Here's how the part is built. I have some questions about the finished solid (model axes, mm). A direction names the side the tool comes from. Coordinates: 2 decimals unless noted, no trailing zeros. Write each loop counter-clockwise with the first axis right and the second up, starting at its lowest first coordinate (ties: lowest second). Pieces come first, ordered by that corner, then holes.
Item 1: For faces 1 (the face through (-20, 2, 0)), 2 (the face through (0, 2, 17.1)), 3 (the face through (20, 2, 0)), which set-ups out of +Z, -Z, +X, -X, +Y, -Y let a thin tool reach every point of the face, with its end or its side?
Item 2: If we section it at C-C (y = 1.5): Please give me the cut outline in (x, z).
Item 3: If we section it at D-D (z = 20): Please give me the cut outline in (x, y), then the cut area to 3 significant figures.
Item 4: If I drill on line 1 (Z direction, x = -10.5, y = 0.75); line 2 (X direction, y = 2.25, z = -9); line 3 (Z direction, x = -7, y = 3.65), over which ranges is the centre line in solid material (lowest first)?
Item 5: If we section it at B-B (z = 15.5): Please give me the cut outline in (x, y).
Item 6: I'm going to push flat-ended pins straight in: pin 1 Ø1.5 at (x, y) = (-2, 2.5) entering from +Z; pin 2 Ø1.5 at (y, z) = (2.5, 8) entering from -X. Where does each tip first touch, or does it pass through?
Item 7: We'd pull the mould along X, two halves only. Please class faces 4 (the face through (1.435, 0.507, 18.504)), 5 (the face through (0, 4, 0)), 6 (the face through (21.5, 0.5, 0.3)): +X half, -X half, draft (parallel to the pull), parting line (faces both ways), or undercut.
Item 8: If we section it at A-A (x = 4.5): Please give me the cut outline in (y, z).
from build123d import *

# Parameters (mm, degrees)
CROQUIS1_W              = 43
CROQUIS1_H              = 45
SALIENTE_EXTRUIR1_DEPTH = 1
CROQUIS2_W              = 40
CROQUIS2_H              = 34
SALIENTE_EXTRUIR2_DEPTH = 3
CROQUIS3_R              = 0.5
CORTAR_EXTRUIR1_DEPTH   = 2


with BuildPart() as part:
    # Croquis1 → Saliente-Extruir1 (new body)
    with BuildSketch(Plane(origin=(0, 0, 0), x_dir=(1, 0, 0), z_dir=(0, 1, 0))):
        Rectangle(CROQUIS1_W, CROQUIS1_H)
    extrude(amount=SALIENTE_EXTRUIR1_DEPTH)

    # Croquis2 → Saliente-Extruir2 (add)
    with BuildSketch(Plane(origin=(0, 1, 0), x_dir=(1, 0, 0), z_dir=(0, 1, 0))):
        with Locations((0, -0.1)):
            Rectangle(CROQUIS2_W, CROQUIS2_H)
    extrude(amount=SALIENTE_EXTRUIR2_DEPTH)

    # Croquis3 → Cortar-Extruir1 (cut, through all)
    with BuildSketch(Plane(origin=(0, 1, 0), x_dir=(1, 0, 0), z_dir=(0, 1, 0))):
        with Locations((1.5, -19)):
            Circle(CROQUIS3_R)
        with Locations((4.5, -19)):
            Circle(CROQUIS3_R)
        with Locations((7.5, -19)):
            Circle(CROQUIS3_R)
        with Locations((10.5, -19)):
            Circle(CROQUIS3_R)
        with Locations((-10.5, -19)):
            Circle(CROQUIS3_R)
        with Locations((-7.5, -19)):
            Circle(CROQUIS3_R)
        with Locations((-4.5, -19)):
            Circle(CROQUIS3_R)
        with Locations((-1.5, -19)):
            Circle(CROQUIS3_R)
    extrude(amount=-CORTAR_EXTRUIR1_DEPTH, mode=Mode.SUBTRACT)


solid = part.part
Answer list:
1. face 1: +Z, -Z, -X, +Y
1. face 2: +Z, +X, -X, +Y
1. face 3: +Z, -Z, +X, +Y
2. outline: (-20, -16.9) - (20, -16.9) - (20, 17.1) - (-20, 17.1) - close
3. outline: (-21.5, 0) - (21.5, 0) - (21.5, 1) - (-21.5, 1) - close
3. area: 43.0 mm2
4. line 1: z = -22.5 to 18.5, 19.5 to 22.5
4. line 2: x = -20 to 20
4. line 3: z = -16.9 to 17.1
5. outline: (-21.5, 0) - (21.5, 0) - (21.5, 1) - (20, 1) - (20, 4) - (-20, 4) - (-20, 1) - (-21.5, 1) - close
6. pin 1: stops at z = 17.1
6. pin 2: stops at x = -20
7. face 4: undercut
7. face 5: draft
7. face 6: +X half
8. outline: (0, -22.5) - (1, -22.5) - (1, -16.9) - (4, -16.9) - (4, 17.1) - (1, 17.1) - (1, 18.5) - (0, 18.5) - close; (0, 19.5) - (1, 19.5) - (1, 22.5) - (0, 22.5) - close
